```python
from build123d import *

# Parameters (mm, degrees)
SKETCH1_W           = 40
SKETCH1_H           = 30
BOSS_EXTRUDE1_DEPTH = 1
SKETCH1_4_W         = 7
SKETCH1_4_H         = 22
BOSS_EXTRUDE2_DEPTH = 1.2
SKETCH2_W           = 5
SKETCH2_H           = 2.5
SKETCH2_W_2         = 2.5
SKETCH2_H_2         = 5
CUT_EXTRUDE15_DEPTH = 0.3
SKETCH3_R           = 1.5
BOSS_EXTRUDE3_DEPTH = 1.8
BOSS_EXTRUDE3_TAPER = 39.5


with BuildPart() as part:
    # Sketch1 → Boss-Extrude1 (new body)
    with BuildSketch(Plane.XY):
        Rectangle(SKETCH1_W, SKETCH1_H)
    extrude(amount=BOSS_EXTRUDE1_DEPTH)

    # Sketch1_4 → Boss-Extrude2 (add)
    with BuildSketch(Plane.XY):
        with Locations((11.166666667, 0)):
            Rectangle(SKETCH1_4_W, SKETCH1_4_H)
    extrude(amount=BOSS_EXTRUDE2_DEPTH)

    # Sketch2 → Cut-Extrude15 (cut)
    with BuildSketch(Plane.XY.offset(1)):
        with Locations((0, -13.75)):
            Rectangle(SKETCH2_W, SKETCH2_H)
        with Locations((-18.75, 0)):
            Rectangle(SKETCH2_W_2, SKETCH2_H_2)
        with Locations((18.75, 0)):
            Rectangle(SKETCH2_W_2, SKETCH2_H_2)
        with Locations((0, 13.75)):
            Rectangle(SKETCH2_W, SKETCH2_H)
    extrude(amount=-CUT_EXTRUDE15_DEPTH, mode=Mode.SUBTRACT)

    # Sketch3 → Boss-Extrude3 (add)
    with BuildSketch(Plane.XY.offset(1.2)):
        with Locations((11.3, -7.75)):
            Circle(SKETCH3_R)
        with Locations((11.3, -3.8)):
            Circle(SKETCH3_R)
        with Locations((11.3, 3.8)):
            Circle(SKETCH3_R)
        with Locations((11.3, 7.75)):
            Circle(SKETCH3_R)
    extrude(amount=BOSS_EXTRUDE3_DEPTH, taper=BOSS_EXTRUDE3_TAPER)


solid = part.part
```
Check sheet for the modelled part. Datum: model origin and axes. Units: mm. A direction names the side the tool comes from. Coordinates: 2 decimals unless noted, no trailing zeros. Loops run counter-clockwise (first coordinate to the right, second up) from the corner with the lowest first, then second, coordinate; pieces in that order, holes last.
1) Access from +Z, -Z, +X, -X, +Y, -Y to the whole of each face (thin tool, end or side, straight path). Record for faces 1 (the face through (0, 14, 0.7)), 2 (the face through (11, 0, 1.2)), 3 (the face through (-19, 0, 0.7)).
2) Sectioned sample at A-A (y = 0). Record the boundary of the cut face in (x, z).
3) Sectioned sample at D-D (y = 10.5). Record the boundary of the cut face in (x, z).
4) Sectioned sample at B-B (x = 1.5). Record the boundary of the cut face in (y, z), and give its area (3 significant figures).
5) Release check for a two-part mould opening along Y. For faces 4 (the face through (0, -14, 0.7)), 5 (the face through (10.99, -3.52, 2.51)), 6 (the face through (-0.3, -15, 0.5)) record: released by +Y, released by -Y, zero draft, split by the parting line, or undercut.
6) Sectioned sample at C-C (z = 1.95). Record the boundary of the cut face in (x, y).
7) Material ranges on probe 1 along Y at (x, z) = (11, 2.3); probe 2 along Y at (x, z) = (11, 2.5); probe 3 along Z at (x, y) = (-18, 7.75), recorded low to high.
8) Gauge pin test, flat ends, axial feed: pin 1 (2 mm diameter, centred on x = 1, y = -14, fed in from +Z); pin 2 (1.5 mm diameter, centred on y = 1, z = 2, fed in from +X); pin 3 (10 mm diameter, centred on x = 10.5, y = 1.5, fed in from -Z); pin 4 (3.5 mm diameter, centred on x = 11.5, y = 2, fed in from +Z). Record the tip position at first contact, or that the pin passes through.
Check sheet entries:
1. face 1: +Z, +Y
1. face 2: +Z
1. face 3: +Z, -X
2. outline: (-20, 0) - (20, 0) - (20, 0.7) - (17.5, 0.7) - (17.5, 1) - (14.67, 1) - (14.67, 1.2) - (7.67, 1.2) - (7.67, 1) - (-17.5, 1) - (-17.5, 0.7) - (-20, 0.7) - close
3. outline: (-20, 0) - (20, 0) - (20, 1) - (14.67, 1) - (14.67, 1.2) - (7.67, 1.2) - (7.67, 1) - (-20, 1) - close
4. outline: (-15, 0) - (15, 0) - (15, 0.7) - (12.5, 0.7) - (12.5, 1) - (-12.5, 1) - (-12.5, 0.7) - (-15, 0.7) - close
4. area: 28.5 mm2
5. face 4: zero draft
5. face 5: undercut
5. face 6: released by -Y
6. outline: circle Ø1.76 at (11.3, -7.75); circle Ø1.76 at (11.3, -3.8); circle Ø1.76 at (11.3, 3.8); circle Ø1.76 at (11.3, 7.75)
7. probe 1: y = -8.26 to -7.24, -4.31 to -3.29, 3.29 to 4.31, 7.24 to 8.26
7. probe 2: y = -8.06 to -7.44, -4.11 to -3.49, 3.49 to 4.11, 7.44 to 8.06
7. probe 3: z = 0 to 1
8. pin 1: stops at z = 0.7
8. pin 2: passes through
8. pin 3: stops at z = 0
8. pin 4: stops at z = 2.95
